from build123d import *

# Parameters (mm, degrees)
F0_R     = 36.71609
F1_DEPTH = 101.6
F0_R_2   = 63.5
F2_DEPTH = 50.8
F3_R     = 5.08
F4_R     = 25.4
F5_DEPTH = 152.4


with BuildPart() as f1:
    # F0 (on Top) → F1 (new body)
    with BuildSketch(Plane.XY):
        Circle(F0_R)
    extrude(amount=F1_DEPTH)

    # F0 (on Top) → F2 (join)
    with BuildSketch(Plane.XY):
        Circle(F0_R_2)
        Circle(F0_R, mode=Mode.SUBTRACT)
        Circle(F0_R)
    extrude(amount=-F2_DEPTH)

    # F3
    f3_edges = [f1.edges().sort_by_distance(p)[0] for p in [
        (-63.5, 0, 0),
        (-63.5, 0, -50.8),
        (-36.71609, 0, 101.6),
    ]]
    fillet(f3_edges, radius=F3_R)

    # F4 (on face) → F5 (cut)
    with BuildSketch(Plane(origin=(0, 0, -50.8), x_dir=(1, 0, 0), z_dir=(0, 0, -1))):
        Circle(F4_R)
    extrude(amount=-F5_DEPTH, mode=Mode.SUBTRACT)


solid = f1.part
For this review, take the finished solid that the model builds, in its own axes (mm). A direction names the side the tool comes from. Give positions to 0.01 mm unless a question says otherwise; leave off trailing zeros. Order: outer loops, then holes, each group sorted by start corner. A loop starts at its lowest first (then second) coordinate and runs counter-clockwise, first axis right, second up. Notation, with made-up numbers: M 13.5,75.25 L 60.5,75.25 A16 ccw 60.5,101.25 Z; hole C -16,-27.5 d2. An arc over 180 degrees is marked long. Answer in a Markdown table with one row per item. Add a question column.
(1) Consider section D-D on z = -27. State the section outline as (x, y) points, and give its area (3 significant figures).
(2) For faces 4 (the face through (-1, -38, 0)), 5 (the face through (25, -12, -50.8)), list the 3-axis set-ups (+Z, -Z, +X, -X, +Y, -Y) from which the entire face can be reached by the end or side of a thin tool; tool diameter is ignored.
(3) Consider section A-A on x = 0. State the section outline as (y, z) points, and give its area (3 significant figures).
(4) Mouldability with a two-part tool opening along Y and no side actions: class faces 1 (the face through (0, 26, 101.6)), 2 (the face through (-5.506, 24.796, 24.333)), 3 (the face through (-13.77, -61.99, -25.12)) as +Y half, -Y half, draft (parallel to the pull), parting line (faces both ways), or undercut.
(5) For pin 1 (10 mm diameter, centred on y = -24.5, z = -18, fed in from -X); pin 2 (10 mm diameter, centred on x = 17, y = -28, fed in from +Z); pin 3 (1.5 mm diameter, centred on y = -2, z = 40.5, fed in from -X); pin 4 (1 mm diameter, centred on x = 28, z = 61, fed in from +Y), all flat-tipped, find the tip position at first contact; note any pin that passes through.
(6) Wall thickness on probe 1 along Y at (x, z) = (0, 50); probe 2 along Z at (x, y) = (-51.5, 5.5); probe 3 along Y at (x, z) = (0, -4): over which ranges is each line inside the solid? List them lowest first. Write a range as [from, to].
(7) Consider section C-C on z = 87.5. State the section outline as (x, y) points.
Evaluation:
| question | item | result |
|---|---|---|
| 1 | outline | C 0,0 d127; hole C 0,0 d50.8 |
| 1 | area | 10,600 mm^2 |
| 2 | face 4 | +Z |
| 2 | face 5 | -Z, +X, -X, +Y, -Y |
| 3 | outline | M -63.5,-45.72 A5.08 ccw -58.42,-50.8 L -25.4,-50.8 L -25.4,101.6 L -31.64,101.6 A5.08 ccw -36.72,96.52 L -36.72,0 L -58.42,0 A5.08 ccw -63.5,-5.08 Z; M 25.4,-50.8 L 58.42,-50.8 A5.08 ccw 63.5,-45.72 L 63.5,-5.08 A5.08 ccw 58.42,0 L 36.72,0 L 36.72,96.52 A5.08 ccw 31.64,101.6 L 25.4,101.6 Z |
| 3 | area | 6,140 mm^2 |
| 4 | face 1 | draft |
| 4 | face 2 | undercut |
| 4 | face 3 | parting line |
| 5 | pin 1 | stops at x = -60.43 |
| 5 | pin 2 | stops at z = 101.6 |
| 5 | pin 3 | stops at x = -36.69 |
| 5 | pin 4 | stops at y = 24.33 |
| 6 | probe 1 | y = [-36.72, -25.4], [25.4, 36.72] |
| 6 | probe 2 | z = [-50.8, 0] |
| 6 | probe 3 | y = [-63.38, -25.4], [25.4, 63.38] |
| 7 | outline | C 0,0 d73.43; hole C 0,0 d50.8 |
